```python
from build123d import *

# Parameters (mm, degrees)
SZKIC1_W                                          = 32
SZKIC1_H                                          = 44.5
DODANIE_WYCI_GNI_CIE1_DEPTH                       = 10
WYTNIJ_WYCI_GNI_CIE1_REACH                        = 31.173
SZKIC2_R                                          = 11.9
WYTNIJ_WYCI_GNI_CIE2_DEPTH                        = 3.4
OTW_R_3_2_3_2_1_D                                 = 3.2
OTW_R_3_2_3_2_1_DEPTH                             = 4
SZKIC7_W                                          = 15
SZKIC7_H                                          = 18
DODANIE_WYCI_GNI_CIE2_DEPTH                       = 5
SFAZOWANIE1_SIZE                                  = 5
SFAZOWANIE2_SIZE                                  = 3
POG_BIENIE_WALCOWE_POD_M3_RUB_Z_BEM_S_D           = 3.6
POG_BIENIE_WALCOWE_POD_M3_RUB_Z_BEM_S_DEPTH       = 24
POG_BIENIE_WALCOWE_POD_M3_RUB_Z_BEM_S_CBORE_D     = 7
POG_BIENIE_WALCOWE_POD_M3_RUB_Z_BEM_S_CBORE_DEPTH = 2.4
POG_BIENIE_WALCOWE_POD_M3_RUB_Z_BEM_S_TIP         = 1.081549114


with BuildPart() as part:
    # Szkic1 → Dodanie-wyciągnięcie1 (new body)
    with BuildSketch(Plane.XY):
        Rectangle(SZKIC1_W, SZKIC1_H)
    extrude(amount=DODANIE_WYCI_GNI_CIE1_DEPTH)

    # Szkic2 → Wytnij-wyciągnięcie1 (cut, up to next)
    with BuildSketch(Plane.XY.offset(10), mode=Mode.PRIVATE) as wytnij_wyci_gni_cie1_sk1:
        with Locations((0, -16.25)):
            Circle(SZKIC2_R)
    wytnij_wyci_gni_cie1_tool1 = extrude(wytnij_wyci_gni_cie1_sk1.sketch, amount=-WYTNIJ_WYCI_GNI_CIE1_REACH, mode=Mode.PRIVATE) & part.part
    add(wytnij_wyci_gni_cie1_tool1.solids().sort_by_distance((0, -16.25, 10))[0], mode=Mode.SUBTRACT)

    # Szkic3 → Wytnij-wyciągnięcie2 (cut)
    with BuildSketch(Plane.XY):
        with BuildLine():
            Line((10.2, -7.3), (10.2, 15.212957385))
            ThreePointArc((10.2, 15.212957385), (9.34039504, 15.618745241), (8.879309367, 16.45))
            Line((8.879309367, 16.45), (-8.879309367, 16.45))
            ThreePointArc((-8.879309367, 16.45), (-9.34039504, 15.618745241), (-10.2, 15.212957385))
            Line((-10.2, 15.212957385), (-10.2, -7.3))
            Line((-10.2, -7.3), (-10.2, -10.120562832))
            Line((-10.2, -10.120562832), (10.2, -10.120562832))
            Line((10.2, -10.120562832), (10.2, -7.3))
        make_face()
    extrude(amount=WYTNIJ_WYCI_GNI_CIE2_DEPTH, mode=Mode.SUBTRACT)

    # Otwór Ø3.2 (3.2)1
    with Locations(Plane(origin=(0, 0, 0), x_dir=(-1, 0, 0), z_dir=(0, 0, -1))):
        with Locations((8, 19.75), (13.5, 14.5), (13.5, 6.5), (13.5, -1.5), (13.5, -9.5), (-13.5, -9.5), (-13.5, -1.5), (-13.5, 6.5), (-13.5, 14.5), (-8, 19.75)):
            Hole(OTW_R_3_2_3_2_1_D / 2, depth=OTW_R_3_2_3_2_1_DEPTH)

    # Szkic7 → Dodanie-wyciągnięcie2 (add)
    with BuildSketch(Plane.XY.offset(10)):
        with Locations((-23.5, -13.25)):
            Rectangle(SZKIC7_W, SZKIC7_H)
    extrude(amount=-DODANIE_WYCI_GNI_CIE2_DEPTH)

    # Sfazowanie1
    sfazowanie1_edges = [part.edges().sort_by_distance(p)[0] for p in [
        (-16, -13.25, 5),
        (-16, -4.25, 7.5),
    ]]
    chamfer(sfazowanie1_edges, length=SFAZOWANIE1_SIZE - 0.0001)  # a hair under: the kernel refuses the full size

    # Sfazowanie2
    sfazowanie2_edges = [part.edges().sort_by_distance(p)[0] for p in [
        (-16, 22.25, 5),
        (16, 22.25, 5),
    ]]
    chamfer(sfazowanie2_edges, length=SFAZOWANIE2_SIZE)

    # Pogłębienie walcowe pod M3 Śrubę z łbem stożkowym ściętym1
    with Locations(Plane(origin=(0, 0, 5), x_dir=(-1, 0, 0), z_dir=(0, 0, -1))):
        with Locations((26, -18.25), (26, -8.25)):
            CounterBoreHole(POG_BIENIE_WALCOWE_POD_M3_RUB_Z_BEM_S_D / 2, POG_BIENIE_WALCOWE_POD_M3_RUB_Z_BEM_S_CBORE_D / 2, POG_BIENIE_WALCOWE_POD_M3_RUB_Z_BEM_S_CBORE_DEPTH, depth=POG_BIENIE_WALCOWE_POD_M3_RUB_Z_BEM_S_DEPTH)
            with Locations((0, 0, -(POG_BIENIE_WALCOWE_POD_M3_RUB_Z_BEM_S_DEPTH + POG_BIENIE_WALCOWE_POD_M3_RUB_Z_BEM_S_TIP / 2))):  # 118° drill point
                Cone(0, POG_BIENIE_WALCOWE_POD_M3_RUB_Z_BEM_S_D / 2, POG_BIENIE_WALCOWE_POD_M3_RUB_Z_BEM_S_TIP, mode=Mode.SUBTRACT)


solid = part.part
```
Verification items for the finished model (mm, model axes). A direction names the side the tool comes from. Coordinates: 2 decimals unless noted, no trailing zeros. Write each loop counter-clockwise with the first axis right and the second up, starting at its lowest first coordinate (ties: lowest second). Pieces come first, ordered by that corner, then holes. Notation, with made-up numbers: (-8, 31) - (20, 31) arc R10 ccw to (20, 46) - close; hole circle Ø10 at (-17.75, 23). An arc over 180 degrees is marked (long way). One line per question, with ' | ' between items. Start each with the question number.
1. Access from +Z, -Z, +X, -X, +Y, -Y to the whole of each face (thin tool, end or side, straight path). Record for faces 4 (the flat face through (0, 6, 3.4)), 5 (the cylindrical face through (11.9, 6.57, 2.03)), 6 (the flat face through (0, 22.25, 5)).
2. Section check A-A (z = 6). Enter the section's corners in (x, y).
3. Gauge pin test, flat ends, axial feed: P1, Ø5, axis at x = -27, y = -10, coming from the -Z side; P2, Ø1, axis at x = 0.5, y = 0.5, coming from the -Z side; P3, Ø1.6, axis at x = 8.5, y = 19.5, coming from the -Z side. Record the tip position at first contact, or that the pin passes through.
4. Material ranges on line 1 along X through (y, z) = (2, 3.25); line 2 along Y through (x, z) = (-13.5, 1.2); line 3 along X through (y, z) = (-7, 6.25), recorded low to high.
5. Section check B-B (y = 11). Enter the section's corners in (x, z).
6. Section check C-C (x = 0). Enter the section's corners in (y, z).
7. Draft check along X on faces 1 (the flat face through (14.52, 20.73, 4.93)), 2 (the cylindrical face through (-15.1, 6.57, 2.03)), 3 (the flat face through (-16, 12, 5)). Enter one of: released by +X, released by -X, zero draft, split by the parting line, or undercut.
8. Section check D-D (x = 8). Enter the section's corners in (y, z).
Computed values:
1) face 4: -Z, -Y | face 5: -Z | face 6: +Z, -Z, +X, -X, +Y
2) outline: (-31, -22.25) - (-10.28, -22.25) arc R11.9 cw (long way) to (10.28, -22.25) - (16, -22.25) - (16, 19.25) - (13, 22.25) - (-13, 22.25) - (-16, 19.25) - (-16, 0.75) - (-21, -4.25) - (-31, -4.25) - close; hole circle Ø7 at (-26, -18.25); hole circle Ø7 at (-26, -8.25)
3) P1: z = 5 | P2: z = 3.4 | P3: z = 4
4) line 1: -16 to -10.2, 10.2 to 16 | line 2: -22.25 to -11.1, -7.9 to -3.1, 0.1 to 4.9, 8.1 to 12.9, 16.1 to 21.75 | line 3: -31 to -29.27, -22.73 to -7.49, 7.49 to 16
5) outline: (-16, 0) - (-10.2, 0) - (-10.2, 3.4) - (10.2, 3.4) - (10.2, 0) - (16, 0) - (16, 10) - (-16, 10) - close
6) outline: (-4.35, 3.4) - (16.45, 3.4) - (16.45, 0) - (22.25, 0) - (22.25, 10) - (-4.35, 10) - close
7) face 1: released by +X | face 2: undercut | face 3: released by -X
8) outline: (-7.44, 3.4) - (16.45, 3.4) - (16.45, 0) - (18.15, 0) - (18.15, 4) - (21.35, 4) - (21.35, 0) - (22.25, 0) - (22.25, 10) - (-7.44, 10) - close
